from build123d import *

# Parameters (mm, degrees)
F1_DEPTH  = 7.5
F3_DEPTH  = 12
F5_DEPTH  = 9
F7_DEPTH  = 13.5
F9_DEPTH  = 10
F11_DEPTH = 12
F13_DEPTH = 9
F15_DEPTH = 13
F17_DEPTH = 10
F19_DEPTH = 12


with BuildPart() as f1:
    # F0 (on Top) → F1 (new body)
    with BuildSketch(Plane.XY):
        Polygon((14.7413760026, 4.7897634128), (0, 15.5), (-14.7413760026, 4.7897634128), (-9.1106714105, -12.5397634128), (9.1106714105, -12.5397634128), align=None)
    extrude(amount=F1_DEPTH)

    # F2 (on Top) → F3 (join)
    with BuildSketch(Plane.XY):
        Polygon((32.9627188236, 4.7897634128), (14.7413760026, 4.7897634128), (9.1106714105, -12.5397634128), (23.8520474131, -23.25), (38.5934234157, -12.5397634128), align=None)
    extrude(amount=F3_DEPTH)

    # F4 (on Top) → F5 (join)
    with BuildSketch(Plane.XY):
        Polygon((14.7413760026, 4.7897634128), (32.9627188236, 4.7897634128), (38.5934234157, 22.1192902384), (23.8520474131, 32.8295268256), (9.1106714105, 22.1192902384), align=None)
    extrude(amount=F5_DEPTH)

    # F6 (on Top) → F7 (join)
    with BuildSketch(Plane.XY):
        Polygon((23.8520474131, 32.8295268256), (38.5934234157, 22.1192902384), (53.3347994183, 32.8295268256), (47.7040948262, 50.1590536512), (29.4827520051, 50.1590536512), align=None)
    extrude(amount=F7_DEPTH)

    # F8 (on Top) → F9 (join)
    with BuildSketch(Plane.XY):
        Polygon((5.630704592, 32.8295268256), (23.8520474131, 32.8295268256), (29.4827520051, 50.1590536512), (14.7413760026, 60.8692902384), (0, 50.1590536512), align=None)
    extrude(amount=F9_DEPTH)

    # F10 (on Top) → F11 (join)
    with BuildSketch(Plane.XY):
        Polygon((-14.7413760026, 60.8692902384), (0, 50.1590536512), (14.7413760026, 60.8692902384), (9.1106714105, 78.1988170641), (-9.1106714105, 78.1988170641), align=None)
    extrude(amount=F11_DEPTH)

    # F12 (on Top) → F13 (join)
    with BuildSketch(Plane.XY):
        Polygon((-23.8520474131, 32.8295268256), (-5.630704592, 32.8295268256), (0, 50.1590536512), (-14.7413760026, 60.8692902384), (-29.4827520051, 50.1590536512), align=None)
    extrude(amount=F13_DEPTH)

    # F14 (on Top) → F15 (join)
    with BuildSketch(Plane.XY):
        Polygon((-53.3347994183, 32.8295268256), (-38.5934234157, 22.1192902384), (-23.8520474131, 32.8295268256), (-29.4827520051, 50.1590536512), (-47.7040948262, 50.1590536512), align=None)
    extrude(amount=F15_DEPTH)

    # F16 (on Top) → F17 (join)
    with BuildSketch(Plane.XY):
        Polygon((-32.9627188236, 4.7897634128), (-14.7413760026, 4.7897634128), (-9.1106714105, 22.1192902384), (-23.8520474131, 32.8295268256), (-38.5934234157, 22.1192902384), align=None)
    extrude(amount=F17_DEPTH)

    # F18 (on Top) → F19 (join)
    with BuildSketch(Plane.XY):
        Polygon((-23.8520474131, -23.25), (-9.1106714105, -12.5397634128), (-14.7413760026, 4.7897634128), (-32.9627188236, 4.7897634128), (-38.5934234157, -12.5397634128), align=None)
    extrude(amount=F19_DEPTH)


solid = f1.part
Can you work these out from the model? Positions are in its coordinate system, mm. A direction names the side the tool comes from. Give positions to 0.01 mm unless a question says otherwise; leave off trailing zeros. Order: outer loops, then holes, each group sorted by start corner. A loop starts at its lowest first (then second) coordinate and runs counter-clockwise, first axis right, second up. Notation, with made-up numbers: M 21.5,-32 L 60.5,-32 A6 ccw 60.5,-24 Z; hole C 54,-29 d1. An arc over 180 degrees is marked long. One line per item, written item: value.
Item 1: If we section it at C-C on y = 6: Write out the boundary of the cut face in (x, z), and give its area (3 significant figures).
Verdict:
outline: M -33.36,0 L -14.35,0 L -14.35,10 L -33.36,10 Z; M -13.08,0 L 13.08,0 L 13.08,7.5 L -13.08,7.5 Z; M 14.35,0 L 33.36,0 L 33.36,9 L 14.35,9 Z
area: 557 mm2
Item 2: For faces 1 (the face through (-16.38, 27.4, 4.93)), 2 (the face through (16.38, -17.82, 5.92)), 3 (the face through (26.7, 41.6, 11.7)), 4 (the face through (-7.474, 55.589, 10.479)), 5 (the face through (-24, 16, 10)), which set-ups out of +Z, -Z, +X, -X, +Y, -Y let a thin tool reach every point of the face, with its end or its side?
Verdict:
face 1: +Z, -Z
face 2: +Z, -Z, -Y
face 3: +Z, +Y
face 4: +Z, -X
face 5: +Z
Item 3: Please list where these lines run through material, in increasing order: line 1 (X direction, y = 7, z = 1.25); line 2 (Z direction, x = -29, y = -6.5); line 3 (Z direction, x = -11, y = -1).
Verdict:
line 1: -33.68 to -14.02, -11.7 to 11.7, 14.02 to 33.68
line 2: 0 to 12
line 3: 0 to 7.5
Item 4: For pin 1 (8 mm diameter, centred on x = 4.5, z = 5.5, fed in from -Y); pin 2 (14 mm diameter, centred on x = 1, y = 7.5, fed in from +Z); pin 3 (10 mm diameter, centred on x = -21, y = -12, fed in from +Z), each with a flat end and sliding along its axis, tell me the tip position at first contact or that it passes through.
Verdict:
pin 1: y = -12.54
pin 2: z = 7.5
pin 3: z = 12
Item 5: If we section it at B-B on y = 18: Write out the boundary of the cut face in (x, z), and give its area (3 significant figures).
Verdict:
outline: M -37.25,0 L -10.45,0 L -10.45,10 L -37.25,10 Z; M 10.45,0 L 37.25,0 L 37.25,9 L 10.45,9 Z
area: 509 mm2
Item 6: If we section it at D-D on x = -31: Write out the boundary of the cut face in (y, z), and give its area (3 significant figures).
Verdict:
outline: M -18.06,0 L 50.16,0 L 50.16,13 L 27.64,13 L 27.64,10 L 4.79,10 L 4.79,12 L -18.06,12 Z
area: 795 mm2
Item 7: If we mould it in two halves opening along Y, with no side actions, what happens to faces 6 (the face through (35.739, 13.333, 4.437)), 7 (the face through (-38, 50.159, 6)), 8 (the face through (-39, 36, 13))? For each: pulls with the +Y half, pulls with the -Y half, needs draft (parallel to the pull), parting line crosses it, or undercut.
Verdict:
face 6: undercut
face 7: pulls with the +Y half
face 8: needs draft
